Design review of the part shown in the three views and the two pictorial views. Dimensions are in mm from the part's minimum x, y and z. Give positions to 0.01 mm unless a question says otherwise; leave off trailing zeros. Write each loop counter-clockwise with the first axis right and the second up, starting at its lowest first coordinate (ties: lowest second). Pieces come first, ordered by that corner, then holes. Notation, with made-up numbers: M -5.75,-8.75 L 21.25,-8.75 A11 cw 21.25,7.25 Z; hole C -1.5,71 d8. An arc over 180 degrees is marked long. Write item = value, one per line.
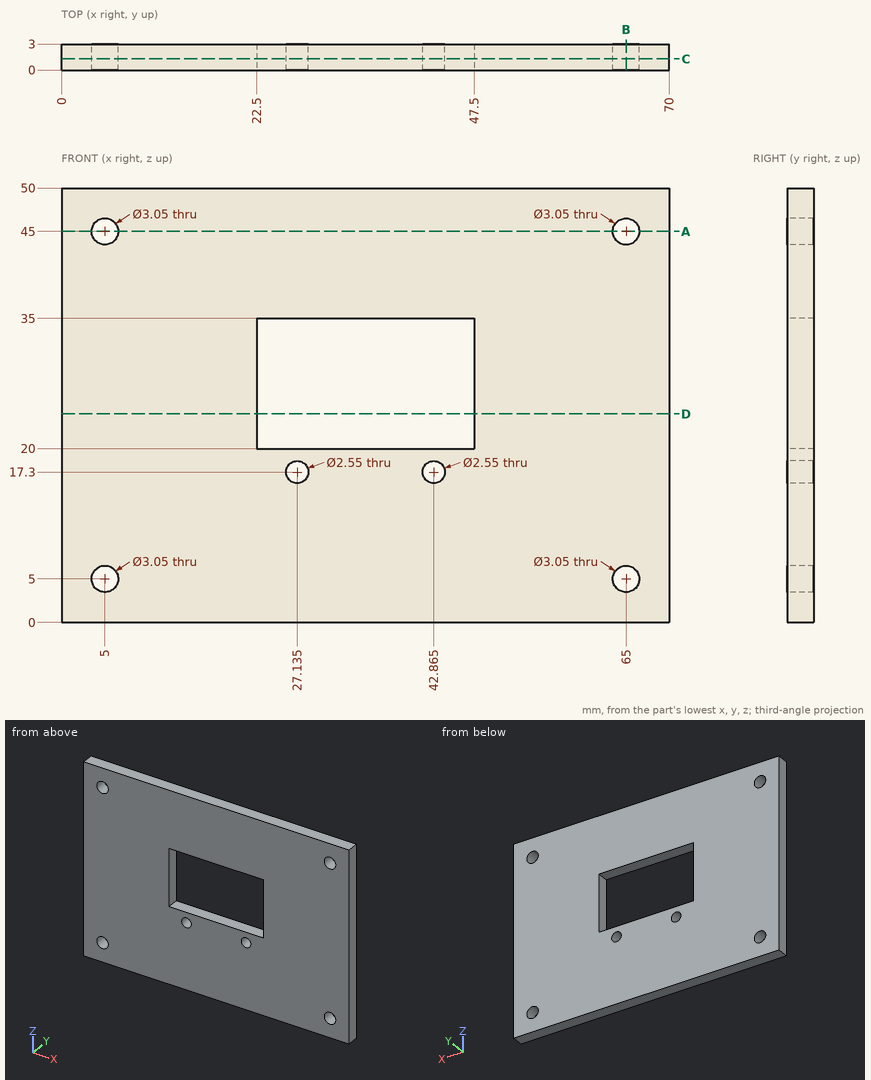
1. For line 1 along X through (y, z) = (2.4, 45) (3 decimals); line 2 along X through (y, z) = (1.5, 17.3); line 3 along Z through (x, y) = (4, 1.75), list the stretches that pass through material, from the lowest coordinate up. Write a range as from..to.
Responses:
line_1 = 0..3.475, 6.525..63.475, 66.525..70
line_2 = 0..25.86, 28.41..41.59, 44.14..70
line_3 = 0..3.85, 6.15..43.85, 46.15..50
2. We need section B-B, the plane x = 65. Write out the cut boundary in (y, z) (3 decimals), then the cut area to 3 significant figures.
Responses:
outline = M 0,0 L 3,0 L 3,3.475 L 0,3.475 Z; M 0,6.525 L 3,6.525 L 3,43.475 L 0,43.475 Z; M 0,46.525 L 3,46.525 L 3,50 L 0,50 Z
area = 132 mm2
3. We need section D-D, the plane z = 24. Write out the cut boundary in (x, y).
Responses:
outline = M 0,0 L 22.5,0 L 22.5,3 L 0,3 Z; M 47.5,0 L 70,0 L 70,3 L 47.5,3 Z
4. Insertion check: P1, Ø2, axis at x = 42.865, z = 17.3, coming from the -Y side. The pin has a flat end and moves straight along its axis. Give the tip position at first contact, or say it passes through.
Responses:
P1 = through
5. We need section C-C, the plane y = 1.3. Write out the cut boundary in (x, z) (3 decimals).
Responses:
outline = M 0,0 L 70,0 L 70,50 L 0,50 Z; hole C 5,5 d3.05; hole C 5,45 d3.05; hole M 22.5,20 L 47.5,20 L 47.5,35 L 22.5,35 Z; hole C 27.135,17.3 d2.55; hole C 42.865,17.3 d2.55; hole C 65,5 d3.05; hole C 65,45 d3.05
6. We need section A-A, the plane z = 45. Write out the cut boundary in (x, y) (3 decimals).
Responses:
outline = M 0,0 L 3.475,0 L 3.475,3 L 0,3 Z; M 6.525,0 L 63.475,0 L 63.475,3 L 6.525,3 Z; M 66.525,0 L 70,0 L 70,3 L 66.525,3 Z
